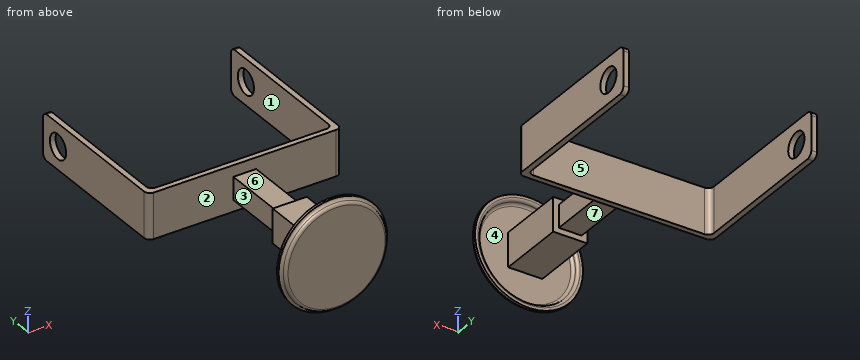
```python
from build123d import *

# Parameters (mm, degrees)
SKETCH3_W           = 38.1
SKETCH3_H           = 38.1
BOSS_EXTRUDE1_DEPTH = 76.2
SKETCH4_W           = 25.4
SKETCH4_H           = 25.4
BOSS_EXTRUDE2_DEPTH = 76.2
BOSS_EXTRUDE3_DEPTH = 25.4
FILLET1_R           = 6.35
FILLET2_R           = 6.35
FILLET3_R           = 6.35
FILLET4_R           = 6.35
SKETCH6_R           = 13.716
CUT_EXTRUDE1_DEPTH  = 402.914443233


with BuildPart() as part:
    # Sketch2 → Revolve1 (revolve)
    with BuildSketch(Plane.XY, mode=Mode.PRIVATE) as revolve1_sk:
        with BuildLine():
            Line((0, 0), (54.261693079, 0))
            ThreePointArc((54.261693079, 0), (56.506757109, 0.92993597), (57.436693079, 3.175))
            ThreePointArc((57.436693079, 3.175), (58.366629049, 5.42006403), (60.611693079, 6.35))
            Line((60.611693079, 6.35), (60.325, 6.35))
            Line((60.325, 6.35), (60.325, 9.525))
            Line((60.325, 9.525), (57.15, 9.525))
            ThreePointArc((57.15, 9.525), (54.90493597, 8.59506403), (53.975, 6.35))
            ThreePointArc((53.975, 6.35), (53.04506403, 4.10493597), (50.8, 3.175))
            Line((50.8, 3.175), (0, 3.175))
            Line((0, 3.175), (0, 0))
        make_face()
    revolve(revolve1_sk.sketch.rotate(Axis((0, 3.175, 0), (0, -1, 0)), 180), axis=Axis((0, 3.175, 0), (0, -1, 0)))

    # Sketch3 → Boss-Extrude1 (add)
    with BuildSketch(Plane(origin=(0, 3.175, 0), x_dir=(1, 0, 0), z_dir=(0, 1, 0))):
        Rectangle(SKETCH3_W, SKETCH3_H)
    extrude(amount=BOSS_EXTRUDE1_DEPTH)

    # Sketch4 → Boss-Extrude2 (add)
    with BuildSketch(Plane(origin=(0, 79.375, 0), x_dir=(1, 0, 0), z_dir=(0, 1, 0))):
        Rectangle(SKETCH4_W, SKETCH4_H)
    extrude(amount=BOSS_EXTRUDE2_DEPTH)

    # Sketch5 → Boss-Extrude3 (add, symmetric)
    with BuildSketch(Plane.XY):
        Polygon((108.077, 155.575), (-108.077, 155.575), (-108.077, 333.375), (-101.727, 333.375), (-101.727, 161.925), (101.727, 161.925), (101.727, 333.375), (108.077, 333.375), align=None)
    extrude(amount=BOSS_EXTRUDE3_DEPTH, both=True)

    # Fillet1
    fillet1_edges = [part.edges().sort_by_distance(p)[0] for p in [
        (101.727, 161.925, 0),
    ]]
    fillet(fillet1_edges, radius=FILLET1_R)

    # Fillet2
    fillet2_edges = [part.edges().sort_by_distance(p)[0] for p in [
        (-101.727, 161.925, 0),
    ]]
    fillet(fillet2_edges, radius=FILLET2_R)

    # Fillet3
    fillet3_edges = [part.edges().sort_by_distance(p)[0] for p in [
        (-108.077, 155.575, 0),
        (108.077, 155.575, 0),
    ]]
    fillet(fillet3_edges, radius=FILLET3_R)

    # Fillet4
    fillet4_edges = [part.edges().sort_by_distance(p)[0] for p in [
        (-104.902, 333.375, -25.4),
        (104.902, 333.375, -25.4),
        (-104.902, 333.375, 25.4),
        (104.902, 333.375, 25.4),
    ]]
    fillet(fillet4_edges, radius=FILLET4_R)

    # Sketch6 → Cut-Extrude1 (cut, through all)
    with BuildSketch(Plane(origin=(108.077, 0, 0), x_dir=(0, 0, -1), z_dir=(1, 0, 0))):
        with Locations((0, 307.975)):
            Circle(SKETCH6_R)
    extrude(amount=-CUT_EXTRUDE1_DEPTH, mode=Mode.SUBTRACT)


solid = part.part
```
Geometry check sheet. Reference: the model listing, model coordinates, mm. Face numbers are marked on the shaded views. A direction names the side the tool comes from. Round coordinates to 2 decimals unless told otherwise and drop trailing zeros. Order: outer loops, then holes, each group sorted by start corner. A loop starts at its lowest first (then second) coordinate and runs counter-clockwise, first axis right, second up. Notation, with made-up numbers: (27.25, -6.5) - (51.25, -6.5) arc R22 cw to (51.25, 3.5) - close; hole circle Ø2 at (9, -4). An arc over 180 degrees is marked (long way). Use a Markdown table: item, result. Add a question column.
(1) Release check for a two-part mould opening along X. For the marked faces 1, 2 and 3 record: pulls with the +X half, pulls with the -X half, needs draft (parallel to the pull), parting line crosses it, or undercut.
(2) Material ranges on line 1 along Y through (x, z) = (42.5, -24) (3 decimals); line 2 along Z through (x, y) = (9, 82.5); line 3 along Y through (x, z) = (16.5, -9.5) (3 decimals), recorded low to high. Write a range as [from, to].
(3) Sectioned sample at B-B, the plane x = 66. Enter the section's corners in (y, z) (3 decimals), and give its area (3 significant figures).
(4) Sectioned sample at C-C, the plane y = 85. Enter the section's corners in (x, z), and give its area (3 significant figures).
(5) Sectioned sample at A-A, the plane y = 260.5. Enter the section's corners in (x, z).
(6) Tool access check on the marked faces 4, 5, 6 and 7. Record the directions out of +Z, -Z, +X, -X, +Y, -Y that give a thin tool (end or side, any length) a straight path to the whole face; none if there is none.
(7) Depth check by flat-ended pin: pin 1 (20.5 mm diameter, centred on y = 106, z = 2.5, fed in from +X); pin 2 (1.5 mm diameter, centred on x = -20, z = -30.5, fed in from -Y); pin 3 (1 mm diameter, centred on x = -46, z = -26.5, fed in from +Y); pin 4 (16.5 mm diameter, centred on y = 307.975, z = 0, fed in from -X). Enter the tip coordinate at first touch or a pass-through.
Answers below:
| question | item | result |
|---|---|---|
| 1 | face 1 | undercut |
| 1 | face 2 | needs draft |
| 1 | face 3 | pulls with the -X half |
| 2 | line 1 | [0, 3.175], [155.575, 161.925] |
| 2 | line 2 | [-12.7, 12.7] |
| 2 | line 3 | [0, 79.375], [155.575, 161.925] |
| 3 | outline | (155.575, -25.4) - (161.925, -25.4) - (161.925, 25.4) - (155.575, 25.4) - close |
| 3 | area | 323 mm² |
| 4 | outline | (-12.7, -12.7) - (12.7, -12.7) - (12.7, 12.7) - (-12.7, 12.7) - close |
| 4 | area | 645 mm² |
| 5 | outline | (-108.08, -25.4) - (-101.73, -25.4) - (-101.73, 25.4) - (-108.08, 25.4) - close; (101.73, -25.4) - (108.08, -25.4) - (108.08, 25.4) - (101.73, 25.4) - close |
| 6 | face 4 | none |
| 6 | face 5 | +Z, -Z, +Y |
| 6 | face 6 | +Z, +X, -X |
| 6 | face 7 | -Z, +X, -X |
| 7 | pin 1 | x = 12.7 |
| 7 | pin 2 | y = 0 |
| 7 | pin 3 | y = 4.83 |
| 7 | pin 4 | through |
